```python
from build123d import *

# Parameters (mm, degrees)
SKETCH_1_W             = 60
SKETCH_1_H             = 40
EXTRUDE_2_DEPTH        = 8
SKETCH_3_R             = 2.25
CUT_EXTRUDE_1_DEPTH    = 8
SKETCH_4_R             = 4
CUT_EXTRUDE_2_DEPTH    = 4.5
SKETCH_5_W             = 7
SKETCH_5_H             = 40
EXTRUDE_3_DEPTH        = 60
CUT_EXTRUDE_3_REACH    = 91.716
SKETCH_6_R             = 2.25
SKETCH_7_R             = 4
CUT_EXTRUDE_4_DEPTH    = 4.5
PATTERN_LINEAR_1_COUNT = 3
PATTERN_LINEAR_1_PITCH = 20


with BuildPart() as part:
    # Sketch 1 → Extrude 2 (new body)
    with BuildSketch(Plane.XY):
        Rectangle(SKETCH_1_W, SKETCH_1_H)
    extrude(amount=EXTRUDE_2_DEPTH)

    # Sketch 3 → Cut-Extrude 1 (cut)
    with BuildSketch(Plane.XY.offset(8)):
        with Locations((15, 12.5)):
            Circle(SKETCH_3_R)
        with Locations((15, -12.5)):
            Circle(SKETCH_3_R)
        with Locations((-10, 12.5)):
            Circle(SKETCH_3_R)
        with Locations((-10, -12.5)):
            Circle(SKETCH_3_R)
    extrude(amount=-CUT_EXTRUDE_1_DEPTH, mode=Mode.SUBTRACT)

    # Sketch 4 → Cut-Extrude 2 (cut)
    with BuildSketch(Plane.XY.offset(8)):
        with Locations((15, 12.5)):
            Circle(SKETCH_4_R)
        with Locations((15, -12.5)):
            Circle(SKETCH_4_R)
        with Locations((-10, 12.5)):
            Circle(SKETCH_4_R)
        with Locations((-10, -12.5)):
            Circle(SKETCH_4_R)
    extrude(amount=-CUT_EXTRUDE_2_DEPTH, mode=Mode.SUBTRACT)

    # Sketch 5 → Extrude 3 (add)
    with BuildSketch(Plane.XY.offset(8)):
        with Locations((-21.5, 0)):
            Rectangle(SKETCH_5_W, SKETCH_5_H)
    extrude(amount=EXTRUDE_3_DEPTH)

    # Sketch 6 → Cut-Extrude 3 (cut, up to next)
    with BuildSketch(Plane.ZY.offset(25), mode=Mode.PRIVATE) as cut_extrude_3_sk1:
        with Locations((63, 10)):
            Circle(SKETCH_6_R)
    cut_extrude_3_tool1 = extrude(cut_extrude_3_sk1.sketch, amount=-CUT_EXTRUDE_3_REACH, mode=Mode.PRIVATE) & part.part
    # Sketch 6 → Cut-Extrude 3 (cut, up to next)
    with BuildSketch(Plane.ZY.offset(25), mode=Mode.PRIVATE) as cut_extrude_3_sk2:
        with Locations((63, -10)):
            Circle(SKETCH_6_R)
    cut_extrude_3_tool2 = extrude(cut_extrude_3_sk2.sketch, amount=-CUT_EXTRUDE_3_REACH, mode=Mode.PRIVATE) & part.part
    cut_extrude_3_1 = cut_extrude_3_tool1.solids().sort_by_distance((-25, 10, 63))[0]
    add(cut_extrude_3_1, mode=Mode.SUBTRACT)
    cut_extrude_3_2 = cut_extrude_3_tool2.solids().sort_by_distance((-25, -10, 63))[0]
    add(cut_extrude_3_2, mode=Mode.SUBTRACT)
    cut_extrude_3 = cut_extrude_3_1 + cut_extrude_3_2  # Cut-Extrude 3 as one shape, for the pattern or mirror that repeats it

    # Sketch 7 → Cut-Extrude 4 (cut)
    with BuildSketch(Plane.ZY.offset(25)):
        with Locations((63, 10)):
            Circle(SKETCH_7_R)
        with Locations((63, -10)):
            Circle(SKETCH_7_R)
    cut_extrude_4 = extrude(amount=-CUT_EXTRUDE_4_DEPTH, mode=Mode.SUBTRACT)

    # Pattern Linear 1: Cut-Extrude 3, Cut-Extrude 4 ×3
    with Locations(*[(0, 0, -i * PATTERN_LINEAR_1_PITCH) for i in range(1, PATTERN_LINEAR_1_COUNT)]):
        add(cut_extrude_3, mode=Mode.SUBTRACT)
        add(cut_extrude_4, mode=Mode.SUBTRACT)

    # Sketch 8 → Loft 2 section 0
    with BuildSketch(Plane.XY.offset(8)):
        with BuildLine():
            Line((-30, 2), (-30, -2))
            Line((-30, -2), (-25, -2))
            Line((-25, -2), (-25, 2))
            Line((-25, 2), (-30, 2))
        make_face()
    # Sketch 9 → Loft 2 section 1
    with BuildSketch(Plane.XY.offset(68)):
        with BuildLine():
            Line((-25, 2), (-26, 2))
            Line((-26, 2), (-26, -2))
            Line((-26, -2), (-25, -2))
            Line((-25, -2), (-25, 2))
        make_face()
    loft()


solid = part.part
```
For this review, take the finished solid that the model builds, in its own axes (mm). A direction names the side the tool comes from. Round coordinates to 2 decimals unless told otherwise and drop trailing zeros. Write each loop counter-clockwise with the first axis right and the second up, starting at its lowest first coordinate (ties: lowest second). Pieces come first, ordered by that corner, then holes. Notation, with made-up numbers: (45.5, -16.75) -> (83.5, -16.75) arc R18 cw to (83.5, 11.25) -> close; hole circle Ø8 at (-21.75, -36). An arc over 180 degrees is marked (long way). One line per question, with ' | ' between items. Start each with the question number.
1) For pin 1 Ø5 at (x, y) = (15, -12.5) entering from +Z; pin 2 Ø2 at (y, z) = (14.5, 31.5) entering from -X; pin 3 Ø9 at (x, y) = (16.5, 12) entering from +Z; pin 4 Ø2.5 at (x, y) = (15, -12.5) entering from -Z, all flat-tipped, find the tip position at first contact; note any pin that passes through.
2) Machinability: for faces 5 (the flat face through (6, 0, 8)), 6 (the flat face through (0, 0, 0)), 7 (the cylindrical face through (-10.521, 16.466, 5.781)), 8 (the flat face through (-20.5, -12, 25)), 9 (the flat face through (-25, -11, 38)), which of the approach directions +Z, -Z, +X, -X, +Y, -Y give a long, thin tool a straight path to every point of the face, cutting with its end or side? Answer none if there is none.
3) Add section A-A (x = -10). Write out the cut boundary in (y, z), and give its area (4 significant figures).
4) Mouldability with a two-part tool opening along Y and no side actions: class faces 1 (the cylindrical face through (-22.782, -11.532, 66.695)), 2 (the flat face through (-20, -20, 21)), 3 (the flat face through (-25, 11, 38)), 4 (the flat face through (-20.5, -12, 65)) as +Y half, -Y half, draft (parallel to the pull), parting line (faces both ways), or undercut.
5) Add section C-C (z = 23). Count the separate pieces of the cut face and the enclosed holes in it, and give its area (4 significant figures).
6) Add section D-D (x = 24). Write out the cut boundary in (y, z).
7) Wall thickness on line 1 along Y through (x, z) = (-10, 0.95); line 2 along Y through (x, z) = (-22, 43); line 3 along Z through (x, y) = (-7, 7): over which ranges is each line inside the solid? List them lowest first.
8) Add section B-B (y = 0.5). Write out the cut boundary in (x, z).
Reported:
1) pin 1: stops at z = 3.5 | pin 2: stops at x = -25 | pin 3: stops at z = 8 | pin 4: passes through
2) face 5: +Z, +X, +Y, -Y | face 6: -Z, +X, -X, +Y, -Y | face 7: +Z | face 8: -X | face 9: +Z, -X, -Y
3) outline: (-20, 0) -> (-14.75, 0) -> (-14.75, 3.5) -> (-16.5, 3.5) -> (-16.5, 8) -> (-20, 8) -> close; (-10.25, 0) -> (10.25, 0) -> (10.25, 3.5) -> (8.5, 3.5) -> (8.5, 8) -> (-8.5, 8) -> (-8.5, 3.5) -> (-10.25, 3.5) -> close; (14.75, 0) -> (20, 0) -> (20, 8) -> (16.5, 8) -> (16.5, 3.5) -> (14.75, 3.5) -> close | area: 216.5 mm²
4) face 1: undercut | face 2: -Y half | face 3: draft | face 4: undercut
5) separate pieces: 3 | enclosed holes: 0 | area: 201.5 mm²
6) outline: (-20, 0) -> (20, 0) -> (20, 8) -> (-20, 8) -> close
7) line 1: y = -20 to -14.75, -10.25 to 10.25, 14.75 to 20 | line 2: y = -20 to -14, -6 to 6, 14 to 20 | line 3: z = 0 to 8
8) outline: (-30, 0) -> (30, 0) -> (30, 8) -> (-18, 8) -> (-18, 68) -> (-26, 68) -> (-30, 8) -> close
